```python
from build123d import *

# Parameters (mm, degrees)
RESSALTO_EXTRUS_O1_DEPTH      = 2.8
RESSALTO_EXTRUS_O1_DEPTH_BACK = 0.15
ESBO_O1_R                     = 3.6
ESBO_O1_R_2                   = 2.45
ESBO_O2_R                     = 2.5
ESBO_O2_R_2                   = 1
RESSALTO_EXTRUS_O2_DEPTH      = 0.5
ESBO_O3_R                     = 3.6
ESBO_O3_R_2                   = 2.45
RESSALTO_EXTRUS_O3_DEPTH      = 2.2
ESBO_O4_W                     = 22
ESBO_O4_H                     = 2.15
RESSALTO_EXTRUS_O4_DEPTH      = 3.6
CORTE_EXTRUS_O2_DEPTH         = 7.2
ESBO_O7_R                     = 2.5
CORTE_EXTRUS_O3_DEPTH         = 2.7
ESBO_O8_R                     = 1.5
ESBO_O8_R_2                   = 0.9
CORTE_EXTRUS_O4_DEPTH         = 6.9
RESSALTO_EXTRUS_O5_DEPTH      = 0.95
CORTE_EXTRUS_O5_DEPTH         = 12
CORTE_EXTRUS_O5_DEPTH_BACK    = 4.95


with BuildPart() as part:
    # Esbo_o1 → Ressalto-extrus_o1 (new, two sides: drawn at the far end of the back side and taken through both)
    with BuildSketch(Plane.XY.offset(-RESSALTO_EXTRUS_O1_DEPTH_BACK)):
        Circle(ESBO_O1_R)
        Circle(ESBO_O1_R_2, mode=Mode.SUBTRACT)
    extrude(amount=RESSALTO_EXTRUS_O1_DEPTH + RESSALTO_EXTRUS_O1_DEPTH_BACK)



with BuildPart() as body_2:
    # Esbo_o2 → Ressalto-extrus_o2 (new body)
    with BuildSketch(Plane(origin=(0, 0, -0.15), x_dir=(-1, 0, 0), z_dir=(0, 0, -1))):
        Circle(ESBO_O2_R)
        Circle(ESBO_O2_R_2, mode=Mode.SUBTRACT)
    extrude(amount=RESSALTO_EXTRUS_O2_DEPTH)


with BuildPart() as part_1:
    add(part.part)

    add(body_2.part)  # Ressalto-extrus_o3 merges body 2
    # Esbo_o3 → Ressalto-extrus_o3 (add)
    with BuildSketch(Plane(origin=(0, 0, -0.15), x_dir=(-1, 0, 0), z_dir=(0, 0, -1))):
        with Locations(Location((0, 0, 0), (0, 0, 180))):
            Circle(ESBO_O3_R)
        with Locations(Location((0, 0, 0), (0, 0, 180))):
            Circle(ESBO_O3_R_2, mode=Mode.SUBTRACT)
    extrude(amount=RESSALTO_EXTRUS_O3_DEPTH)

    # Esbo_o4 → Ressalto-extrus_o4 (add, symmetric)
    with BuildSketch(Plane(origin=(0, 0, 0), x_dir=(1, 0, 0), z_dir=(0, 1, 0))):
        with Locations((-7.325, 0.315)):
            Rectangle(ESBO_O4_W, ESBO_O4_H)
    extrude(amount=RESSALTO_EXTRUS_O4_DEPTH, both=True)

    # Esbo_o5 → Corte-extrus_o2 (cut)
    with BuildSketch(Plane.XY.offset(0.76)):
        with BuildLine():
            ThreePointArc((0, -3.6), (-0.28434443, -3.588753021), (-0.566912184, -3.555082358))
            Line((-0.566912184, -3.555082358), (-16.183639111, -2.317736326))
            ThreePointArc((-16.183639111, -2.317736326), (-17.70771571, -1.577761723), (-18.325, -1.7e-08))
            Line((-18.325, -1.7e-08), (-18.325, -3.6))
            Line((-18.325, -3.6), (0, -3.6))
        make_face()
        with BuildLine():
            ThreePointArc((0, 3.6), (3.6, 0), (0, -3.6))
            Line((0, -3.6), (3.675, -3.6))
            Line((3.675, -3.6), (3.675, 3.6))
            Line((3.675, 3.6), (0, 3.6))
        make_face()
        with BuildLine():
            Line((-16.183639111, 2.317736326), (-0.566912184, 3.555082358))
            ThreePointArc((-0.566912184, 3.555082358), (-0.28434443, 3.588753021), (0, 3.6))
            Line((0, 3.6), (-18.325, 3.6))
            Line((-18.325, 3.6), (-18.325, -1.7e-08))
            ThreePointArc((-18.325, -1.7e-08), (-17.707715722, 1.57776171), (-16.183639111, 2.317736326))
        make_face()
    extrude(amount=-CORTE_EXTRUS_O2_DEPTH, mode=Mode.SUBTRACT)

    # Esbo_o7 → Corte-extrus_o3 (cut)
    with BuildSketch(Plane.XY.offset(2.8)):
        Circle(ESBO_O7_R)
    extrude(amount=-CORTE_EXTRUS_O3_DEPTH, mode=Mode.SUBTRACT)

    # Esbo_o8 → Corte-extrus_o4 (cut, symmetric)
    with BuildSketch(Plane.XY.offset(0.1)):
        Circle(ESBO_O8_R)
        with Locations((-6, 0)):
            Circle(ESBO_O8_R_2)
        with Locations((-8.5, 0)):
            Circle(ESBO_O8_R_2)
        with Locations((-11, 0)):
            Circle(ESBO_O8_R_2)
        with Locations((-13.5, 0)):
            Circle(ESBO_O8_R_2)
        with Locations((-16, 0)):
            Circle(ESBO_O8_R_2)
    extrude(amount=CORTE_EXTRUS_O4_DEPTH, both=True, mode=Mode.SUBTRACT)

    # Esbo_o10 → Ressalto-extrus_o5 (add)
    with BuildSketch(Plane(origin=(0, 0, -1.39), x_dir=(-1, 0, 0), z_dir=(0, 0, -1))):
        with BuildLine():
            Line((0.566912184, -3.555082358), (5.1, -3.195916302))
            Line((5.1, -3.195916302), (5.1, -2.395916302))
            Line((5.1, -2.395916302), (2.686928558, -2.395916302))
            ThreePointArc((2.686928558, -2.395916302), (1.727074515, -3.158672763), (0.566912184, -3.555082358))
        make_face()
        with BuildLine():
            ThreePointArc((3.577708764, 0.4), (3.6, 0), (3.577708764, -0.4))
            Line((3.577708764, -0.4), (5.193774225, -0.4))
            ThreePointArc((5.193774225, -0.4), (5.1, 0), (5.193774225, 0.4))
            Line((5.193774225, 0.4), (3.577708764, 0.4))
        make_face()
        with BuildLine():
            ThreePointArc((0.566912184, 3.555082358), (1.727074515, 3.158672763), (2.686928558, 2.395916302))
            Line((2.686928558, 2.395916302), (5.1, 2.395916302))
            Line((5.1, 2.395916302), (5.1, 3.195916302))
            Line((5.1, 3.195916302), (0.566912184, 3.555082358))
        make_face()
    extrude(amount=RESSALTO_EXTRUS_O5_DEPTH)

    # Esbo_o11 → Corte-extrus_o5 (cut, two sides: drawn at the far end of the back side and taken through both)
    with BuildSketch(Plane(origin=(0, 0, 0), x_dir=(1, 0, 0), z_dir=(0, 1, 0)).offset(-CORTE_EXTRUS_O5_DEPTH_BACK)):
        Polygon((-5.1, 1.39), (-2.045555334, 3.15348445), (-5.859008957, 3.15348445), (-5.859008957, 1.39), align=None)
    extrude(amount=CORTE_EXTRUS_O5_DEPTH + CORTE_EXTRUS_O5_DEPTH_BACK, mode=Mode.SUBTRACT)


solid = part_1.part
```
Input: part model. Units: mm. Frame: model coordinates. A direction names the side the tool comes from. Give positions to 0.01 mm unless a question says otherwise; leave off trailing zeros. Order: outer loops, then holes, each group sorted by start corner. A loop starts at its lowest first (then second) coordinate and runs counter-clockwise, first axis right, second up. Notation, with made-up numbers: M -8,-3 L 38,-3 A24 cw 38,10 Z; hole C 7.25,21 d11. An arc over 180 degrees is marked long. Return JSON: item names as keys, results as strings.
Item 1: Cut plane A-A (z = -0.2). Return loops of the section in (x, y) (3 decimals), then the cut area to 3 significant figures.
Solutions:
{"outline": "M -16.184,-2.318 L -0.567,-3.555 A3.6 ccw long -0.567,3.555 L -16.184,2.318 A2.325 ccw Z; hole C -16,0 d1.8; hole C -13.5,0 d1.8; hole C -11,0 d1.8; hole C -8.5,0 d1.8; hole C -6,0 d1.8; hole C 0,0 d3", "area": "104 mm^2"}
Item 2: Cut plane B-B (x = -11). Return loops of the section in (y, z), then the cut area to 3 significant figures.
Solutions:
{"outline": "M -2.73,-1.39 L -0.9,-1.39 L -0.9,0.76 L -2.73,0.76 Z; M 0.9,-1.39 L 2.73,-1.39 L 2.73,0.76 L 0.9,0.76 Z", "area": "7.86 mm^2"}
Item 3: First-contact query: P1, Ø2, axis at x = -16, y = 0, coming from the +Z side; P2, Ø2.5, axis at x = -11, y = 0, coming from the -Z side; P3, Ø4, axis at x = -1, y = 0.5, coming from the +Z side; P4, Ø0.8, axis at x = -4, z = -2, coming from the -Y side. Flat tips, straight axial feed; report the tip coordinate or a pass-through.
Solutions:
{"P1": "z = 0.76", "P2": "z = -1.39", "P3": "z = 2.8", "P4": "y = -3.31"}
Item 4: Cut plane C-C (z = 0.95). Return loops of the section in (x, y).
Solutions:
{"outline": "C 0,0 d7.2; hole C 0,0 d5"}
Item 5: Ray query, probe 1 along Z at (x, y) = (-10, -2.75); probe 2 along Y at (x, z) = (-6, -0.4); probe 3 along Y at (x, z) = (0, -1.9). Return the intervals inside material, ascending.
Solutions:
{"probe 1": "-1.39 to 0.76", "probe 2": "-3.12 to -0.9, 0.9 to 3.12", "probe 3": "-3.6 to -2.45, 2.45 to 3.6"}
Item 6: Cut plane D-D (x = -6). Return loops of the section in (y, z).
Solutions:
{"outline": "M -3.12,-1.39 L -0.9,-1.39 L -0.9,0.76 L -3.12,0.76 Z; M 0.9,-1.39 L 3.12,-1.39 L 3.12,0.76 L 0.9,0.76 Z"}
Item 7: Pull-direction query (Y, two-part tool) for faces 1 (the flat face through (-3, 3, -2.34)), 2 (the cylindrical face through (-1.5, 0.07, -0.63)); classes: +Y half, -Y half, draft (parallel to the pull), parting line (faces both ways), or undercut.
Solutions:
{"face 1": "draft", "face 2": "undercut"}
Item 8: Access query for faces 3 (the flat face through (-4.2, -0.4, -1.7)), 4 (the flat face through (2, 0, -1.39)), 5 (the flat face through (-0.9, 2.5, 2.8)), 6 (the flat face through (0, -2, 0.1)). Directions: +Z, -Z, +X, -X, +Y, -Y. A direction counts if a zero-diameter tool reaches every point of the face in a straight line with its end or side. Return the directions, or none.
Solutions:
{"face 3": "-Z, -X", "face 4": "-Z", "face 5": "+Z, +X, -X, +Y, -Y", "face 6": "+Z"}
